Source: CAD feature listing. Evaluate the final solid. Frame: model axes, mm. A direction names the side the tool comes from. Round coordinates to 2 decimals unless told otherwise and drop trailing zeros. Write each loop counter-clockwise with the first axis right and the second up, starting at its lowest first coordinate (ties: lowest second). Pieces come first, ordered by that corner, then holes. Notation, with made-up numbers: M 19.5,2 L 74.5,2 A24 ccw 74.5,27 Z; hole C 86,2.25 d6. An arc over 180 degrees is marked long. Use a Markdown table: item, result.
```python
from build123d import *

# Parameters (mm, degrees)
SKETCH_1_W          = 32.2
SKETCH_1_H          = 10.1
EXTRUDE_1_DEPTH     = 5.8
CUT_EXTRUDE_1_DEPTH = 1
SKETCH_3_R          = 0.25
EXTRUDE_2_DEPTH     = 2
SKETCH_4_R          = 0.5
SKETCH_4_R_2        = 0.524489224
SKETCH_4_W          = 0.85
SKETCH_4_H          = 3.2
SKETCH_4_W_2        = 2.3
SKETCH_4_H_2        = 0.85
CUT_EXTRUDE_2_DEPTH = 0.2


with BuildPart() as part:
    # Эскиз1 → Бобышка-Вытянуть1 (new body)
    with BuildSketch(Plane(origin=(0, 0, 0), x_dir=(1, 0, 0), z_dir=(0, 1, 0))):
        Rectangle(SKETCH_1_W, SKETCH_1_H)
    extrude(amount=EXTRUDE_1_DEPTH)

    # Эскиз2 → Вырез-Вытянуть1 (cut)
    with BuildSketch(Plane.XZ):
        Polygon((-16.1, 3.55), (-14.6, 3.55), (-14.6, 5.05), (14.6, 5.05), (14.6, 3.55), (16.1, 3.55), (16.1, -3.55), (14.6, -3.55), (14.6, -5.05), (-14.6, -5.05), (-14.6, -3.55), (-16.1, -3.55), align=None)
    extrude(amount=-CUT_EXTRUDE_1_DEPTH, mode=Mode.SUBTRACT)

    # Эскиз3 → Бобышка-Вытянуть2 (add)
    with BuildSketch(Plane.XZ.offset(-1)):
        with Locations((-6.35, 3.81)):
            Circle(SKETCH_3_R)
        with Locations((-3.81, 3.81)):
            Circle(SKETCH_3_R)
        with Locations((-1.27, 3.81)):
            Circle(SKETCH_3_R)
        with Locations((1.27, 3.81)):
            Circle(SKETCH_3_R)
        with Locations((3.81, 3.81)):
            Circle(SKETCH_3_R)
        with Locations((6.35, 3.81)):
            Circle(SKETCH_3_R)
        with Locations((-3.81, -3.81)):
            Circle(SKETCH_3_R)
        with Locations((-1.27, -3.81)):
            Circle(SKETCH_3_R)
        with Locations((1.27, -3.81)):
            Circle(SKETCH_3_R)
        with Locations((3.81, -3.81)):
            Circle(SKETCH_3_R)
        with Locations((6.35, -3.81)):
            Circle(SKETCH_3_R)
        with Locations((-6.35, -3.81)):
            Circle(SKETCH_3_R)
    extrude(amount=EXTRUDE_2_DEPTH)

    # Эскиз4 → Вырез-Вытянуть2 (cut)
    with BuildSketch(Plane(origin=(0, 5.8, 0), x_dir=(1, 0, 0), z_dir=(0, 1, 0))):
        with Locations((0, 2.088518093)):
            Circle(SKETCH_4_R)
        with Locations((-8.994155163, -2.922635465)):
            Circle(SKETCH_4_R)
        with Locations((-0.009676216, -1.263887704)):
            Circle(SKETCH_4_R_2)
        with Locations((-0.919099914, -2.922635465)):
            Circle(SKETCH_4_R_2)
        with Locations((14.988407473, -2.922635465)):
            Circle(SKETCH_4_R_2)
        with Locations((7.017698273, -2.922635465)):
            Circle(SKETCH_4_R_2)
        with Locations((-13.773526097, -1.311481907)):
            Rectangle(SKETCH_4_W, SKETCH_4_H)
        with Locations((-12, 3.260742105)):
            Rectangle(SKETCH_4_W_2, SKETCH_4_H_2)
        with Locations((-13.775, 2.088518093)):
            Rectangle(SKETCH_4_W, SKETCH_4_H)
        with Locations((-10.225, 2.077364535)):
            Rectangle(SKETCH_4_W, SKETCH_4_H)
        with Locations((-10.213082834, -1.322635465)):
            Rectangle(SKETCH_4_W, SKETCH_4_H)
        with Locations((-12, 0.368523253)):
            Rectangle(SKETCH_4_W_2, SKETCH_4_H_2)
        with Locations((-11.998526097, -2.488527153)):
            Rectangle(SKETCH_4_W_2, SKETCH_4_H_2)
        with Locations((-5.773526097, -1.311481907)):
            Rectangle(SKETCH_4_W, SKETCH_4_H)
        with Locations((-4, 3.260742105)):
            Rectangle(SKETCH_4_W_2, SKETCH_4_H_2)
        with Locations((-5.775, 2.088518093)):
            Rectangle(SKETCH_4_W, SKETCH_4_H)
        with Locations((-2.225, 2.077364535)):
            Rectangle(SKETCH_4_W, SKETCH_4_H)
        with Locations((-2.213082834, -1.322635465)):
            Rectangle(SKETCH_4_W, SKETCH_4_H)
        with Locations((-4, 0.368523253)):
            Rectangle(SKETCH_4_W_2, SKETCH_4_H_2)
        with Locations((-3.998526097, -2.488527153)):
            Rectangle(SKETCH_4_W_2, SKETCH_4_H_2)
        with Locations((2.226473903, -1.311481907)):
            Rectangle(SKETCH_4_W, SKETCH_4_H)
        with Locations((4, 3.260742105)):
            Rectangle(SKETCH_4_W_2, SKETCH_4_H_2)
        with Locations((2.225, 2.088518093)):
            Rectangle(SKETCH_4_W, SKETCH_4_H)
        with Locations((5.775, 2.077364535)):
            Rectangle(SKETCH_4_W, SKETCH_4_H)
        with Locations((5.786917166, -1.322635465)):
            Rectangle(SKETCH_4_W, SKETCH_4_H)
        with Locations((4, 0.368523253)):
            Rectangle(SKETCH_4_W_2, SKETCH_4_H_2)
        with Locations((4.001473903, -2.488527153)):
            Rectangle(SKETCH_4_W_2, SKETCH_4_H_2)
        with Locations((10.226473903, -1.311481907)):
            Rectangle(SKETCH_4_W, SKETCH_4_H)
        with Locations((12, 3.260742105)):
            Rectangle(SKETCH_4_W_2, SKETCH_4_H_2)
        with Locations((10.225, 2.088518093)):
            Rectangle(SKETCH_4_W, SKETCH_4_H)
        with Locations((13.775, 2.077364535)):
            Rectangle(SKETCH_4_W, SKETCH_4_H)
        with Locations((13.786917166, -1.322635465)):
            Rectangle(SKETCH_4_W, SKETCH_4_H)
        with Locations((12, 0.368523253)):
            Rectangle(SKETCH_4_W_2, SKETCH_4_H_2)
        with Locations((12.001473903, -2.488527153)):
            Rectangle(SKETCH_4_W_2, SKETCH_4_H_2)
    extrude(amount=-CUT_EXTRUDE_2_DEPTH, mode=Mode.SUBTRACT)


solid = part.part
```
Q1. Mould query, pull axis X, two halves, no side actions, for faces 1 (the flat face through (-15.3, 0.5, -3.55)), 2 (the flat face through (12, 5.6, 2.5)). Classes: +X half, -X half, draft (parallel to the pull), parting line (faces both ways), or undercut.
Results are:
| item | result |
|---|---|
| face 1 | draft |
| face 2 | undercut |
Q2. Section A-A on y = 0.5. Give the number of separate pieces and of enclosed holes in the cut face, plus the area to 3 significant figures.
Results are:
| item | result |
|---|---|
| separate pieces | 16 |
| enclosed holes | 0 |
| area | 11.4 mm^2 |
Q3. First-contact query: pin 1 Ø3 at (x, z) = (-1, 2) entering from -Y. Flat tip, straight axial feed; report the tip coordinate or a pass-through.
Results are:
| item | result |
|---|---|
| pin 1 | y = 1 |
Q4. Section B-B on x = -7.5. Return loops of the section in (y, z), plus the area to 3 significant figures.
Results are:
| item | result |
|---|---|
| outline | M 1,-5.05 L 5.8,-5.05 L 5.8,5.05 L 1,5.05 Z |
| area | 48.5 mm^2 |
Q5. Reachability of faces 3 (the flat face through (15.3, 0.5, 3.55)), 4 (the flat face through (-4, 5.6, -3)), 5 (the flat face through (-15, 0, 4)), 6 (the flat face through (-4, 5.8, 1)) from +Z, -Z, +X, -X, +Y, -Y: full face, straight path, thin tool, end or side. Return the list, or none.
Results are:
| item | result |
|---|---|
| face 3 | +X, -X, -Y |
| face 4 | +Y |
| face 5 | +Z, -Z, -X, -Y |
| face 6 | +Z, -Z, +X, -X, +Y |
Q6. Line query: L1, parallel to Z at x = 0, y = 5.7; L2, parallel to Y at x = -4, z = 4.25; L3, parallel to Z at x = 15, y = 0.75. Output: solid intervals per line, ascending.
Results are:
| item | result |
|---|---|
| L1 | -5.05 to -2.59, -1.59 to 0.74, 1.79 to 5.05 |
| L2 | 1 to 5.8 |
| L3 | -5.05 to -3.55, 3.55 to 5.05 |
